Autodesk Inventor part; units mm, degrees
ref_plane "YZ Plane" through (0, 0, 0) normal (1, 0, 0) x (0, 1, 0)
ref_plane "XZ Plane" through (0, 0, 0) normal (0, 1, 0) x (-1, 0, 0)
ref_plane "XY Plane" through (0, 0, 0) normal (0, 0, 1) x (1, 0, 0)
sketch "スケッチ1" plane through (0, 0, 0) normal (0, 0, 1) x (1, 0, 0)
  line L0 (10, -10) -> (-10, -10)
  line L1 (-10, -10) -> (-10, 10)
  line L2 (-10, 10) -> (10, 10)
  line L3 (10, 10) -> (10, -10)
  line L4 (10, -10) -> (-10, 10) construction
  line L5 (-10, -10) -> (10, 10) construction
  line L6 (9, 9) -> (-9, 9)
  line L7 (-9, 9) -> (-9, -9)
  line L8 (-9, -9) -> (9, -9)
  line L9 (9, -9) -> (9, 9)
  point P0 (0, 0)
  dimension "d0" = 20
  dimension "d1" = 20
  dimension "d2" = 1
extrude "押し出し1" add sketch "スケッチ1" along normal blind 465
sketch "スケッチ2" plane through (10, -10, 0) normal (1, 0, 0) x (0, 0, -1)
  line L0 (0, 10) -> (-465, 10)
  line L1 (-465, 0) -> (-465, 20)
  line L2 (0, 0) -> (0, 20)
  point P0 (-403, 10)
  point P1 (-60, 10)
  point P2 (-10, 10)
  point P3 (-453, 10)
  point P4 (-82.5, 10)
  point P5 (-232.5, 10)
  dimension "d5" = 343
  dimension "d6" = 50
  dimension "d7" = 10
  dimension "d15" = 50
  dimension "d17" = 465
  dimension "d28" = 150
hole "穴1" at (10, 0, 403) at (10, 0, 60) at (10, 0, 10) at (10, 0, 453) at (10, 0, 82.5) direction (-1, 0, 0) diameter 3.3 end through all
sketch "スケッチ3" plane through (-10, 10, 0) normal (0, 1, 0) x (1, 0, 0)
  line L0 (10, 0) -> (10, -465)
  line L1 (20, -465) -> (0, -465)
  point P0 (10, -242.5)
  point P1 (10, -222.5)
  point P2 (10, -232.5)
  dimension "d19" = 20
  dimension "d20" = 10
hole "穴2" at (0, 10, 242.5) at (0, 10, 222.5) direction (0, -1, 0) diameter 3.3 end through all
sketch "スケッチ4" plane through (0, 0, 0) normal (0, 0, -1) x (-1, 0, 0)
  line L0 (-10, 10) -> (10, 10)
  line L1 (-10, -10) -> (-10, 10)
  line L2 (10, -10) -> (-10, -10)
  line L3 (10, 10) -> (10, -10)
  line L4 (-9, 9) -> (-9, -9)
  line L5 (9, 9) -> (-9, 9)
  line L6 (9, -9) -> (9, 9)
  line L7 (-9, -9) -> (9, -9)
  point P0 (0, 0)
extrude "押し出し2" add sketch "スケッチ4" along normal blind 70
sketch "スケッチ5" plane through (-10, 10, 465) normal (0, 1, 0) x (1, 0, 0)
  line L0 (10, 465) -> (10, 535)
  line L1 (1, 535) -> (19, 535)
  circle A0 centre (10, 475) radius 2.5
  circle A1 centre (10, 525) radius 2.5
  circle A2 centre (10, 489) radius 2.5
  circle A3 centre (10, 511) radius 2.5
  circle A4 centre (10, 500) radius 6
  dimension "d34" = 5
  dimension "d35" = 5
  dimension "d38" = 5
  dimension "d39" = 5
  dimension "d40" = 22
  dimension "d42" = 12
  dimension "d43" = 25
  dimension "d44" = 25
  dimension "d45" = 11
  dimension "d46" = 35
  dimension "d47" = 60
extrude "押し出し3" cut sketch "スケッチ5" against normal blind 70
equation "\"d35\" = d38"
equation "\"d39\" = d38"
equation "\"d45\" = 0.5 * d40"
properties part number "kaku_1010_530"
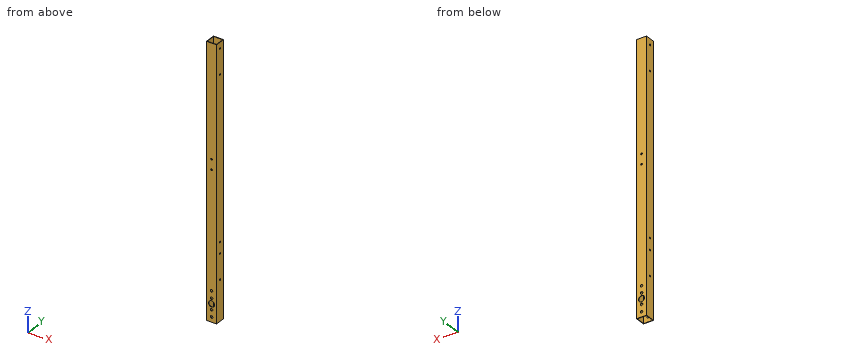
Work out the finished part from the listing and answer in its coordinate system (mm). Give positions to 0.01 mm unless a question says otherwise; leave off trailing zeros. Loops run counter-clockwise (first coordinate to the right, second up) from the corner with the lowest first, then second, coordinate; pieces in that order, holes last. Notation, with made-up numbers: (71, -3) - (109, -3) arc R19 cw to (109, 17) - close; hole circle Ø7 at (4, -27). An arc over 180 degrees is marked (long way). Answer in a Markdown table with one row per item. Add a question column.
Q1. Consider line 1 along Z through (x, y) = (9.8, 0); line 2 along Y through (x, z) = (-4.5, 428); line 3 along X through (y, z) = (-9.45, -46). Determine where each line is inside the solid, lowest interval first.
Q2. The part is cut by section B-B (y = 5.75). Determine the outline of the cut face in (x, z), and give its area (3 significant figures).
Q3. The part is cut by section C-C (z = 413). Determine the outline of the cut face in (x, y).
Q4. The part is cut by section A-A (z = -35). Determine the outline of the cut face in (x, y).
Q5. Each of these flat-tipped pins is pushed along its axis until it touches: P1, Ø4, axis at y = 0, z = 82.5, coming from the -X side; P2, Ø2, axis at y = 0, z = 453, coming from the -X side. Where does it stop, or does it pass through?
Solution:
| question | item | result |
|---|---|---|
| 1 | line 1 | z = -70 to 8.35, 11.65 to 58.35, 61.65 to 80.85, 84.15 to 401.35, 404.65 to 451.35, 454.65 to 465 |
| 1 | line 2 | y = -10 to -9, 9 to 10 |
| 1 | line 3 | x = -10 to -2.5, 2.5 to 10 |
| 2 | outline | (-10, -70) - (-9, -70) - (-9, 465) - (-10, 465) - close; (9, -70) - (10, -70) - (10, 465) - (9, 465) - close |
| 2 | area | 1,070 mm² |
| 3 | outline | (-10, -10) - (10, -10) - (10, 10) - (-10, 10) - close; hole (-9, -9) - (9, -9) - (9, 9) - (-9, 9) - close |
| 4 | outline | (-10, -10) - (-6, -10) - (-6, -9) - (-9, -9) - (-9, 9) - (-6, 9) - (-6, 10) - (-10, 10) - close; (6, -10) - (10, -10) - (10, 10) - (6, 10) - (6, 9) - (9, 9) - (9, -9) - (6, -9) - close |
| 5 | P1 | stops at x = -10 |
| 5 | P2 | passes through |
